Read the model definition and answer for the solid it produces. Units are mm, in the model's axes. Coordinates: 2 decimals unless noted, no trailing zeros. Write each loop counter-clockwise with the first axis right and the second up, starting at its lowest first coordinate (ties: lowest second). Pieces come first, ordered by that corner, then holes. Notation, with made-up numbers: (39.25, -29.5) -> (77.25, -29.5) arc R9 cw to (77.25, -23.5) -> close; hole circle Ø4 at (-9, -31). An arc over 180 degrees is marked (long way). One line per item, written item: value. Start each with the question number.
1. Find section C-C, the plane x = 25. Write down the section's boundary in (y, z).
2. Find section A-A, the plane y = -38. Write down the section's boundary in (x, z), and give its area (3 significant figures).
3. Find section B-B, the plane z = 1.8. Write down the section's boundary in (x, y), and give its area (3 significant figures).
4. Given P1, Ø2, axis at x = 2, z = 1.5, coming from the +Y side; P2, Ø0.6, axis at y = 1.5, z = 4.5, coming from the -X side; P3, Ø1.6, axis at y = -12.5, z = 4, coming from the -X side, each flat-ended and moving along its own axis, determine where each tip first touches the part or whether it passes through.
5. For a pull along X with two mould halves and no side action, classify faces 1 (the cylindrical face through (49.478, 15.019, 1.528)), 2 (the flat face through (1, 1, 0)), 3 (the flat face through (1, 1, 3.1)) as pulls with the +X half, pulls with the -X half, needs draft (parallel to the pull), parting line crosses it, or undercut.
6. Consider line 1 along X through (y, z) = (-31.5, 4.75); line 2 along X through (y, z) = (-41, 3.3); line 3 along Z through (x, y) = (-21, -19.5). Determine where each line is inside the solid, lowest interval first.
```python
from build123d import *

# Parameters (mm, degrees)
F0_R         = 50
F1_DEPTH     = 3.1
F2_W         = 1.5
F2_H         = 92
F2_H_2       = 72
F2_H_3       = 52
F2_H_4       = 32
F2_H_5       = 12
F2_W_2       = 1.3582831621
F2_H_6       = 17.2204319388
F3_DEPTH     = 2
F4_T1_DEPTH  = 11.5
F4_T3_DEPTH  = 11.5
F4_T5_DEPTH  = 21.5
F4_T10_DEPTH = 21.5
F4_T15_DEPTH = 21.5
F4_T20_DEPTH = 21.5
F4_T25_DEPTH = 21.5
F4_T30_DEPTH = 21.5
F4_T35_DEPTH = 21.5
F4_T40_DEPTH = 21.5
F4_T45_DEPTH = 21.5
F4_T50_DEPTH = 21.3582831621
F4_T55_DEPTH = 21.3582831621


# Not quite as in the source:
# - a fillet or chamfer that OpenCascade refuses, or shapes differently, is made with other operations: its cross-section is extruded or revolved along the edge and cut away or added


with BuildPart() as f1:
    # F0 (on Top) → F1 (new body)
    with BuildSketch(Plane.XY):
        with Locations((1.7865982372, 0)):
            Circle(F0_R)
    extrude(amount=F1_DEPTH)

    # F2 (on face) → F3 (join)
    with BuildSketch(Plane.XY.offset(3.1)):
        Rectangle(F2_W, F2_H)
        with Locations((-10, 0)):
            Rectangle(F2_W, F2_H_2)
        with Locations((-20, 0)):
            Rectangle(F2_W, F2_H_3)
        with Locations((-30, 0)):
            Rectangle(F2_W, F2_H_4)
        with Locations((-40, 0)):
            Rectangle(F2_W, F2_H_5)
        with Locations((10, 0)):
            Rectangle(F2_W, F2_H_2)
        with Locations((20, 0)):
            Rectangle(F2_W, F2_H_3)
        with Locations((30, 0)):
            Rectangle(F2_W_2, F2_H_6)
    extrude(amount=F3_DEPTH)

    # F4: fillet of radius 5 on 16 edges, made by hand

    # F4_s2 → F4_t1 (cut)
    with BuildSketch(Plane.YZ.offset(9.25)):
        with BuildLine():
            ThreePointArc((-36, 3.1), (-34.2360679775, 4.572135955), (-32, 5.1))
            Line((-32, 5.1), (-36, 5.1))
            Line((-36, 5.1), (-36, 3.1))
        make_face()
        with BuildLine():
            ThreePointArc((36, 3.1), (34.2360679775, 4.572135955), (32, 5.1))
            Line((32, 5.1), (36, 5.1))
            Line((36, 5.1), (36, 3.1))
        make_face()
    extrude(amount=F4_T1_DEPTH, mode=Mode.SUBTRACT)

    # F4_s4 → F4_t3 (cut)
    with BuildSketch(Plane.YZ.offset(19.25)):
        with BuildLine():
            ThreePointArc((26, 3.1), (24.2360679775, 4.572135955), (22, 5.1))
            Line((22, 5.1), (26, 5.1))
            Line((26, 5.1), (26, 3.1))
        make_face()
        with BuildLine():
            ThreePointArc((-26, 3.1), (-24.2360679775, 4.572135955), (-22, 5.1))
            Line((-22, 5.1), (-26, 5.1))
            Line((-26, 5.1), (-26, 3.1))
        make_face()
    extrude(amount=F4_T3_DEPTH, mode=Mode.SUBTRACT)

    # F4_s6 → F4_t5 (cut)
    with BuildSketch(Plane.YZ.offset(-10.75)):
        with BuildLine():
            ThreePointArc((46, 3.1), (44.2360679775, 4.572135955), (42, 5.1))
            Line((42, 5.1), (46, 5.1))
            Line((46, 5.1), (46, 3.1))
        make_face()
        with BuildLine():
            ThreePointArc((-46, 3.1), (-44.2360679775, 4.572135955), (-42, 5.1))
            Line((-42, 5.1), (-46, 5.1))
            Line((-46, 5.1), (-46, 3.1))
        make_face()
    extrude(amount=F4_T5_DEPTH, mode=Mode.SUBTRACT)


with BuildPart() as f4_tool8:
    # F4_s9 → F4_t10 (new body)
    with BuildSketch(Plane.YZ.offset(0.75)):
        with BuildLine():
            ThreePointArc((36, 3.1), (34.2360679775, 4.572135955), (32, 5.1))
            Line((32, 5.1), (36, 5.1))
            Line((36, 5.1), (36, 3.1))
        make_face()
    extrude(amount=-F4_T10_DEPTH)

    split(bisect_by=Plane.YZ.offset(-0.75), keep=Keep.BOTTOM)


with BuildPart() as f1_1:
    add(f1.part)

    # F4_t7: cut F4_tool8
    add(f4_tool8.part, mode=Mode.SUBTRACT)


with BuildPart() as f4_tool13:
    # F4_s14 → F4_t15 (new body)
    with BuildSketch(Plane.YZ.offset(-9.25)):
        with BuildLine():
            ThreePointArc((26, 3.1), (24.2360679775, 4.572135955), (22, 5.1))
            Line((22, 5.1), (26, 5.1))
            Line((26, 5.1), (26, 3.1))
        make_face()
    extrude(amount=-F4_T15_DEPTH)

    split(bisect_by=Plane.YZ.offset(-10.75), keep=Keep.BOTTOM)


with BuildPart() as f1_2:
    add(f1_1.part)

    # F4_t12: cut F4_tool13
    add(f4_tool13.part, mode=Mode.SUBTRACT)


with BuildPart() as f4_tool18:
    # F4_s19 → F4_t20 (new body)
    with BuildSketch(Plane.YZ.offset(-19.25)):
        with BuildLine():
            ThreePointArc((16, 3.1), (14.2360679775, 4.572135955), (12, 5.1))
            Line((12, 5.1), (16, 5.1))
            Line((16, 5.1), (16, 3.1))
        make_face()
    extrude(amount=-F4_T20_DEPTH)

    split(bisect_by=Plane.YZ.offset(-20.75), keep=Keep.BOTTOM)


with BuildPart() as f1_3:
    add(f1_2.part)

    # F4_t17: cut F4_tool18
    add(f4_tool18.part, mode=Mode.SUBTRACT)


with BuildPart() as f4_tool23:
    # F4_s24 → F4_t25 (new body)
    with BuildSketch(Plane.YZ.offset(-29.25)):
        with BuildLine():
            ThreePointArc((6, 3.1), (4.2360679775, 4.572135955), (2, 5.1))
            Line((2, 5.1), (6, 5.1))
            Line((6, 5.1), (6, 3.1))
        make_face()
    extrude(amount=-F4_T25_DEPTH)

    split(bisect_by=Plane.YZ.offset(-30.75), keep=Keep.BOTTOM)


with BuildPart() as f1_4:
    add(f1_3.part)

    # F4_t22: cut F4_tool23
    add(f4_tool23.part, mode=Mode.SUBTRACT)


with BuildPart() as f4_tool28:
    # F4_s29 → F4_t30 (new body)
    with BuildSketch(Plane.YZ.offset(-50.75)):
        with BuildLine():
            ThreePointArc((-6, 3.1), (-4.2360679775, 4.572135955), (-2, 5.1))
            Line((-2, 5.1), (-6, 5.1))
            Line((-6, 5.1), (-6, 3.1))
        make_face()
    extrude(amount=F4_T30_DEPTH)

    split(bisect_by=Plane.YZ.offset(-30.75), keep=Keep.BOTTOM)


with BuildPart() as f1_5:
    add(f1_4.part)

    # F4_t27: cut F4_tool28
    add(f4_tool28.part, mode=Mode.SUBTRACT)


with BuildPart() as f4_tool33:
    # F4_s34 → F4_t35 (new body)
    with BuildSketch(Plane.YZ.offset(-40.75)):
        with BuildLine():
            ThreePointArc((-16, 3.1), (-14.2360679775, 4.572135955), (-12, 5.1))
            Line((-12, 5.1), (-16, 5.1))
            Line((-16, 5.1), (-16, 3.1))
        make_face()
    extrude(amount=F4_T35_DEPTH)

    split(bisect_by=Plane.YZ.offset(-20.75), keep=Keep.BOTTOM)


with BuildPart() as f1_6:
    add(f1_5.part)

    # F4_t32: cut F4_tool33
    add(f4_tool33.part, mode=Mode.SUBTRACT)


with BuildPart() as f4_tool38:
    # F4_s39 → F4_t40 (new body)
    with BuildSketch(Plane.YZ.offset(-30.75)):
        with BuildLine():
            ThreePointArc((-26, 3.1), (-24.2360679775, 4.572135955), (-22, 5.1))
            Line((-22, 5.1), (-26, 5.1))
            Line((-26, 5.1), (-26, 3.1))
        make_face()
    extrude(amount=F4_T40_DEPTH)

    split(bisect_by=Plane.YZ.offset(-10.75), keep=Keep.BOTTOM)


with BuildPart() as f1_7:
    add(f1_6.part)

    # F4_t37: cut F4_tool38
    add(f4_tool38.part, mode=Mode.SUBTRACT)


with BuildPart() as f4_tool43:
    # F4_s44 → F4_t45 (new body)
    with BuildSketch(Plane.YZ.offset(-20.75)):
        with BuildLine():
            ThreePointArc((-36, 3.1), (-34.2360679775, 4.572135955), (-32, 5.1))
            Line((-32, 5.1), (-36, 5.1))
            Line((-36, 5.1), (-36, 3.1))
        make_face()
    extrude(amount=F4_T45_DEPTH)

    split(bisect_by=Plane.YZ.offset(-0.75), keep=Keep.BOTTOM)


with BuildPart() as f1_8:
    add(f1_7.part)

    # F4_t42: cut F4_tool43
    add(f4_tool43.part, mode=Mode.SUBTRACT)


with BuildPart() as f4_tool48:
    # F4_s49 → F4_t50 (new body)
    with BuildSketch(Plane.YZ.offset(19.3208584189)):
        with BuildLine():
            ThreePointArc((-8.6102159694, 3.1), (-6.8462839469, 4.572135955), (-4.6102159694, 5.1))
            Line((-4.6102159694, 5.1), (-8.6102159694, 5.1))
            Line((-8.6102159694, 5.1), (-8.6102159694, 3.1))
        make_face()
    extrude(amount=F4_T50_DEPTH)

    split(bisect_by=Plane.YZ.offset(20.75), keep=Keep.TOP)


with BuildPart() as f1_9:
    add(f1_8.part)

    # F4_t47: cut F4_tool48
    add(f4_tool48.part, mode=Mode.SUBTRACT)


with BuildPart() as f4_tool53:
    # F4_s54 → F4_t55 (new body)
    with BuildSketch(Plane.YZ.offset(40.6791415811)):
        with BuildLine():
            ThreePointArc((8.6102159694, 3.1), (6.8462839469, 4.572135955), (4.6102159694, 5.1))
            Line((4.6102159694, 5.1), (8.6102159694, 5.1))
            Line((8.6102159694, 5.1), (8.6102159694, 3.1))
        make_face()
    extrude(amount=-F4_T55_DEPTH)

    split(bisect_by=Plane.YZ.offset(20.75), keep=Keep.TOP)


with BuildPart() as f1_10:
    add(f1_9.part)

    # F4_t52: cut F4_tool53
    add(f4_tool53.part, mode=Mode.SUBTRACT)


solid = f1_10.part
```
Answer block:
1. outline: (-44.28, 0) -> (44.28, 0) -> (44.28, 3.1) -> (-44.28, 3.1) -> close
2. outline: (-30.71, 0) -> (34.28, 0) -> (34.28, 3.1) -> (0.75, 3.1) -> (0.75, 5.1) -> (-0.75, 5.1) -> (-0.75, 3.1) -> (-30.71, 3.1) -> close
2. area: 204 mm2
3. outline: circle Ø100 at (1.79, 0)
3. area: 7,850 mm2
4. P1: stops at y = 50
4. P2: stops at x = -40.75
4. P3: stops at x = -30.75
5. face 1: parting line crosses it
5. face 2: needs draft
5. face 3: undercut
6. line 1: x = -10.75 to -9.25, -0.75 to 0.75, 9.25 to 10.75
6. line 2: x = -0.75 to 0.75
6. line 3: z = 0 to 3.1
